from build123d import *

# Parameters (mm, degrees)
F0_W     = 50.8
F0_H     = 25.4
F0_W_2   = 47.625
F0_H_2   = 22.225
F1_DEPTH = 101.6
F2_R     = 2.5527
F3_DEPTH = 25.4
F4_R     = 2.5527
F5_DEPTH = 50.801
F6_R     = 4.7625
F7_DEPTH = 3.175


with BuildPart() as f1:
    # F0 (on Top) → F1 (new body)
    with BuildSketch(Plane.XY):
        Rectangle(F0_W, F0_H)
        Rectangle(F0_W_2, F0_H_2, mode=Mode.SUBTRACT)
    extrude(amount=F1_DEPTH)

    # F2 (on face) → F3 (cut)
    with BuildSketch(Plane.XZ.offset(12.7)):
        with Locations((-12.7, 12.7)):
            Circle(F2_R)
        with Locations((-12.7, 38.1)):
            Circle(F2_R)
        with Locations((-12.7, 63.5)):
            Circle(F2_R)
        with Locations((-12.7, 88.9)):
            Circle(F2_R)
        with Locations((12.7, 12.7)):
            Circle(F2_R)
        with Locations((12.7, 38.1)):
            Circle(F2_R)
        with Locations((12.7, 63.5)):
            Circle(F2_R)
        with Locations((12.7, 88.9)):
            Circle(F2_R)
    extrude(amount=-F3_DEPTH, mode=Mode.SUBTRACT)

    # F4 (on face) → F5 (cut, through all)
    with BuildSketch(Plane(origin=(-25.4, 0, 0), x_dir=(0, -1, 0), z_dir=(-1, 0, 0))):
        with Locations((0, 88.9)):
            Circle(F4_R)
        with Locations((0, 63.5)):
            Circle(F4_R)
        with Locations((0, 38.1)):
            Circle(F4_R)
        with Locations((0, 12.7)):
            Circle(F4_R)
    extrude(amount=-F5_DEPTH, mode=Mode.SUBTRACT)

    # F6 (on face) → F7 (cut)
    with BuildSketch(Plane(origin=(-25.4, 0, 0), x_dir=(0, -1, 0), z_dir=(-1, 0, 0))):
        with Locations((0, 12.7)):
            Circle(F6_R)
        with Locations((0, 38.1)):
            Circle(F6_R)
    extrude(amount=-F7_DEPTH, mode=Mode.SUBTRACT)


solid = f1.part
The listing builds one solid part. Answer for the finished solid, in the listing's coordinates (mm). A direction names the side the tool comes from. Give positions to 0.01 mm unless a question says otherwise; leave off trailing zeros. Loops run counter-clockwise (first coordinate to the right, second up) from the corner with the lowest first, then second, coordinate; pieces in that order, holes last. Notation, with made-up numbers: (10, 52) - (18, 52) arc R29 ccw to (18, 78) - close; hole circle Ø6 at (-12, 75). An arc over 180 degrees is marked (long way). Write each question's results on one line, items separated by ' | '.
1. Find section A-A, the plane y = -6. Write down the section's boundary in (x, z), then the cut area to 3 significant figures.
Resolved:
outline: (-25.4, 0) - (-23.81, 0) - (-23.81, 101.6) - (-25.4, 101.6) - close; (23.81, 0) - (25.4, 0) - (25.4, 101.6) - (23.81, 101.6) - close | area: 323 mm^2
2. A flat-ended cylindrical pin translates along its axis: P1, Ø10, axis at x = 8.5, y = -1.5, coming from the +Z side. Find the tip coordinate at first contact, or state that the pin passes through.
Resolved:
P1: passes through
3. Which of the six approach directions +Z, -Z, +X, -X, +Y, -Y give full straight-line access (tool end or side, diameter ignored) to faces 4 (the face through (-24.617, -2.198, 33.875)), 5 (the face through (-11.522, 11.895, 86.635))?
Resolved:
face 4: -X | face 5: +Y, -Y
4. Find section D-D, the plane z = 52.5. Write down the section's boundary in (x, y), then the cut area to 3 significant figures.
Resolved:
outline: (-25.4, -12.7) - (25.4, -12.7) - (25.4, 12.7) - (-25.4, 12.7) - close; hole (-23.81, -11.11) - (23.81, -11.11) - (23.81, 11.11) - (-23.81, 11.11) - close | area: 232 mm^2
5. Find section C-C, the plane z = 12.7. Count the separate pieces of the cut face and the enclosed holes in it, then the cut area to 3 significant figures.
Resolved:
separate pieces: 6 | enclosed holes: 0 | area: 176 mm^2
6. Find section B-B, the plane x = 20. Write down the section's boundary in (y, z).
Resolved:
outline: (-12.7, 0) - (-11.11, 0) - (-11.11, 101.6) - (-12.7, 101.6) - close; (11.11, 0) - (12.7, 0) - (12.7, 101.6) - (11.11, 101.6) - close
7. Consider probe 1 along Z at (x, y) = (-24.6, 0); probe 2 along Z at (x, y) = (12.7, 11.85); probe 3 along X at (y, z) = (-9.5, 91.5). Determine where each line is inside the solid, lowest interval first. Write a range as from..to.
Resolved:
probe 1: z = 0..7.94, 17.46..33.34, 42.86..60.95, 66.05..86.35, 91.45..101.6 | probe 2: z = 0..10.15, 15.25..35.55, 40.65..60.95, 66.05..86.35, 91.45..101.6 | probe 3: x = -25.4..-23.81, 23.81..25.4
8. For a pull along X with two mould halves and no side action, classify faces 1 (the face through (-25.4, 0, 50)), 2 (the face through (13.878, 11.895, 86.635)), 3 (the face through (0, -12.7, 50)) as +X half, -X half, draft (parallel to the pull), parting line (faces both ways), or undercut.
Resolved:
face 1: -X half | face 2: undercut | face 3: draft
